Could you check a few things on this model? Use its own coordinates, in mm. Coordinates: 2 decimals unless noted, no trailing zeros. Order: outer loops, then holes, each group sorted by start corner. A loop starts at its lowest first (then second) coordinate and runs counter-clockwise, first axis right, second up. Notation, with made-up numbers: (51.25, 68) - (77.25, 68) arc R14 cw to (77.25, 82) - close; hole circle Ø10 at (75, 4.5). An arc over 180 degrees is marked (long way). One line per item, written item: value.
from build123d import *

# Parameters (mm, degrees)
SKETCH1_W           = 34.29
SKETCH1_H           = 276.86
SKETCH1_W_2         = 6.35
SKETCH1_H_2         = 3.175
BOSS_EXTRUDE1_DEPTH = 3.175
SKETCH3_W           = 2.54
SKETCH3_H           = 3.175
CUT_EXTRUDE1_DEPTH  = 490.020092379
SKETCH4_W           = 2.54
SKETCH4_H           = 6.35
SKETCH4_W_2         = 3.175
SKETCH4_H_2         = 13.97
CUT_EXTRUDE2_DEPTH  = 490.020092379


with BuildPart() as part:
    # Sketch1 → Boss-Extrude1 (new body)
    with BuildSketch(Plane(origin=(0, 0, 0), x_dir=(1, 0, 0), z_dir=(0, 1, 0))):
        with Locations((17.145, 138.43)):
            Rectangle(SKETCH1_W, SKETCH1_H)
        with Locations((51.435, 138.43)):
            Rectangle(SKETCH1_W, SKETCH1_H)
        Polygon((34.29, 403.86), (34.29, 276.86), (68.58, 276.86), (74.93, 276.86), (62.865, 403.86), (56.515, 403.86), align=None)
        Polygon((-6.35, 276.86), (0, 276.86), (34.29, 276.86), (34.29, 403.86), (12.065, 403.86), (5.715, 403.86), align=None)
        Polygon((12.065, 403.86), (34.29, 403.86), (56.515, 403.86), (56.515, 480.06), (50.165, 480.06), (43.815, 480.06), (24.765, 480.06), (18.415, 480.06), (12.065, 480.06), align=None)
        with Locations((21.59, 481.6475)):
            Rectangle(SKETCH1_W_2, SKETCH1_H_2)
        with Locations((46.99, 481.6475)):
            Rectangle(SKETCH1_W_2, SKETCH1_H_2)
    extrude(amount=BOSS_EXTRUDE1_DEPTH)

    # Sketch3 → Cut-Extrude1 (cut, through all)
    with BuildSketch(Plane(origin=(0, 3.175, 0), x_dir=(1, 0, 0), z_dir=(0, 1, 0))):
        with Locations((1.27, 20.6375)):
            Rectangle(SKETCH3_W, SKETCH3_H)
        with Locations((67.31, 20.6375)):
            Rectangle(SKETCH3_W, SKETCH3_H)
        with Locations((1.27, 131.7625)):
            Rectangle(SKETCH3_W, SKETCH3_H)
        with Locations((67.31, 131.7625)):
            Rectangle(SKETCH3_W, SKETCH3_H)
    extrude(amount=-CUT_EXTRUDE1_DEPTH, mode=Mode.SUBTRACT)

    # Sketch4 → Cut-Extrude2 (cut, through all)
    with BuildSketch(Plane(origin=(0, 3.175, 0), x_dir=(1, 0, 0), z_dir=(0, 1, 0))):
        with Locations((29.845, 3.175)):
            Rectangle(SKETCH4_W, SKETCH4_H)
        with Locations((32.7025, 3.175)):
            Rectangle(SKETCH4_W_2, SKETCH4_H)
        with Locations((35.8775, 3.175)):
            Rectangle(SKETCH4_W_2, SKETCH4_H)
        with Locations((38.735, 3.175)):
            Rectangle(SKETCH4_W, SKETCH4_H)
        with Locations((35.8775, 13.335)):
            Rectangle(SKETCH4_W_2, SKETCH4_H_2)
        with Locations((32.7025, 13.335)):
            Rectangle(SKETCH4_W_2, SKETCH4_H_2)
    extrude(amount=-CUT_EXTRUDE2_DEPTH, mode=Mode.SUBTRACT)


solid = part.part
Item 1: I'm going to push flat-ended pins straight in: pin 1 Ø1.6 at (y, z) = (2, -236) entering from +X; pin 2 Ø1 at (x, y) = (35.5, 1) entering from +Z; pin 3 Ø1.6 at (y, z) = (2, -481) entering from -X (3 decimals). Where does each tip first touch, or does it pass through?
Conclusion:
pin 1: x = 68.58
pin 2: z = -20.32
pin 3: x = 18.415
Item 2: I want a section at A-A on z = -444. Please give me the cut outline in (x, y) (3 decimals), then the cut area to 3 significant figures.
Conclusion:
outline: (12.065, 0) - (56.515, 0) - (56.515, 3.175) - (12.065, 3.175) - close
area: 141 mm²
Item 3: If I drill on probe 1 along Z at (x, y) = (54, 0.25); probe 2 along X at (y, z) = (0.35, -52); probe 3 along Z at (x, y) = (37, 2.2), over which ranges is the centre line in solid material (lowest first)?
Conclusion:
probe 1: -480.06 to 0
probe 2: 0 to 68.58
probe 3: -480.06 to -20.32
Item 4: I want a section at B-B on z = -158. Please give me the cut outline in (x, y) (3 decimals).
Conclusion:
outline: (0, 0) - (68.58, 0) - (68.58, 3.175) - (0, 3.175) - close
